Geometry check sheet. Reference: the model listing, model coordinates, mm. Round coordinates to 2 decimals unless told otherwise and drop trailing zeros. Order: outer loops, then holes, each group sorted by start corner. A loop starts at its lowest first (then second) coordinate and runs counter-clockwise, first axis right, second up. Notation, with made-up numbers: (15, 85) - (30, 85) arc R29 cw to (30, 118) - close; hole circle Ø3 at (-5, -23.5). An arc over 180 degrees is marked (long way). Use a Markdown table: item, result. Add a question column.
(1) Section check B-B on y = -0.2. Record the boundary of the cut face in (x, z), then the cut area to 3 significant figures.
(2) Thickness scan on line 1 along Z through (x, y) = (0, 1.3); line 2 along X through (y, z) = (-0.1, 21); line 3 along X through (y, z) = (0.6, 31). Record the ranges inside material, lowest first. Write a range as [from, to].
(3) Section check C-C on x = 0. Record the boundary of the cut face in (y, z), then the cut area to 4 significant figures.
(4) Gauge pin test, flat end, axial feed: P1, Ø1.8, axis at x = 0, z = 30, coming from the +Y side. Record the tip position at first contact, or that the pin passes through.
(5) Mould release check, pull along X, two halves, no side actions. Record for faces 1 (the face through (0, 1, 0)), 2 (the face through (6.5, 0, 19.7)), 3 (the face through (0.195, 0.031, 31.487)), 4 (the face through (-6.5, 0, 19.7)): released by +X, released by -X, zero draft, split by the parting line, or undercut.
(6) Section check A-A on z = 30. Record the boundary of the cut face in (x, y).
(7) Section check D-D on y = 1.6. Record the boundary of the cut face in (x, z).
```python
from build123d import *

# Parameters (mm, degrees)
RESSALTO_EXTRUS_O1_DEPTH = 40
CORTE_EXTRUS_O1_REACH    = 43.192
ESBO_O2_R                = 1.5


with BuildPart() as part:
    # Esboço1 → Ressalto-extrusão1 (new body)
    with BuildSketch(Plane.XY):
        Polygon((-8.75, 2.25), (8.75, 2.25), (4.25, -2.25), (-4.25, -2.25), align=None)
    extrude(amount=RESSALTO_EXTRUS_O1_DEPTH)

    # Esboço2 → Corte-extrusão1 (cut, up to next)
    with BuildSketch(Plane(origin=(0, 2.25, 0), x_dir=(1, 0, 0), z_dir=(0, 1, 0)), mode=Mode.PRIVATE) as corte_extrus_o1_sk1:
        with Locations(Location((0, -20, 0), (0, 0, 180))):
            Circle(ESBO_O2_R)
    corte_extrus_o1_tool1 = extrude(corte_extrus_o1_sk1.sketch, amount=-CORTE_EXTRUS_O1_REACH, mode=Mode.PRIVATE) & part.part
    # Esboço2 → Corte-extrusão1 (cut, up to next)
    with BuildSketch(Plane(origin=(0, 2.25, 0), x_dir=(1, 0, 0), z_dir=(0, 1, 0)), mode=Mode.PRIVATE) as corte_extrus_o1_sk2:
        with Locations(Location((0, -10, 0), (0, 0, 180))):
            Circle(ESBO_O2_R)
    corte_extrus_o1_tool2 = extrude(corte_extrus_o1_sk2.sketch, amount=-CORTE_EXTRUS_O1_REACH, mode=Mode.PRIVATE) & part.part
    # Esboço2 → Corte-extrusão1 (cut, up to next)
    with BuildSketch(Plane(origin=(0, 2.25, 0), x_dir=(1, 0, 0), z_dir=(0, 1, 0)), mode=Mode.PRIVATE) as corte_extrus_o1_sk3:
        with Locations(Location((0, -30, 0), (0, 0, 180))):
            Circle(ESBO_O2_R)
    corte_extrus_o1_tool3 = extrude(corte_extrus_o1_sk3.sketch, amount=-CORTE_EXTRUS_O1_REACH, mode=Mode.PRIVATE) & part.part
    add(corte_extrus_o1_tool1.solids().sort_by_distance((0, 2.25, 20))[0], mode=Mode.SUBTRACT)
    add(corte_extrus_o1_tool2.solids().sort_by_distance((0, 2.25, 10))[0], mode=Mode.SUBTRACT)
    add(corte_extrus_o1_tool3.solids().sort_by_distance((0, 2.25, 30))[0], mode=Mode.SUBTRACT)


solid = part.part
```
Check sheet entries:
| question | item | result |
|---|---|---|
| 1 | outline | (-6.3, 0) - (6.3, 0) - (6.3, 40) - (-6.3, 40) - close; hole circle Ø3 at (0, 10); hole circle Ø3 at (0, 20); hole circle Ø3 at (0, 30) |
| 1 | area | 483 mm2 |
| 2 | line 1 | z = [0, 8.5], [11.5, 18.5], [21.5, 28.5], [31.5, 40] |
| 2 | line 2 | x = [-6.4, -1.12], [1.12, 6.4] |
| 2 | line 3 | x = [-7.1, -1.12], [1.12, 7.1] |
| 3 | outline | (-2.25, 0) - (2.25, 0) - (2.25, 8.5) - (-2.25, 8.5) - close; (-2.25, 11.5) - (2.25, 11.5) - (2.25, 18.5) - (-2.25, 18.5) - close; (-2.25, 21.5) - (2.25, 21.5) - (2.25, 28.5) - (-2.25, 28.5) - close; (-2.25, 31.5) - (2.25, 31.5) - (2.25, 40) - (-2.25, 40) - close |
| 3 | area | 139.5 mm2 |
| 4 | P1 | passes through |
| 5 | face 1 | zero draft |
| 5 | face 2 | released by +X |
| 5 | face 3 | undercut |
| 5 | face 4 | released by -X |
| 6 | outline | (-8.75, 2.25) - (-4.25, -2.25) - (-1.5, -2.25) - (-1.5, 2.25) - close; (1.5, -2.25) - (4.25, -2.25) - (8.75, 2.25) - (1.5, 2.25) - close |
| 7 | outline | (-8.1, 0) - (8.1, 0) - (8.1, 40) - (-8.1, 40) - close; hole circle Ø3 at (0, 10); hole circle Ø3 at (0, 20); hole circle Ø3 at (0, 30) |
